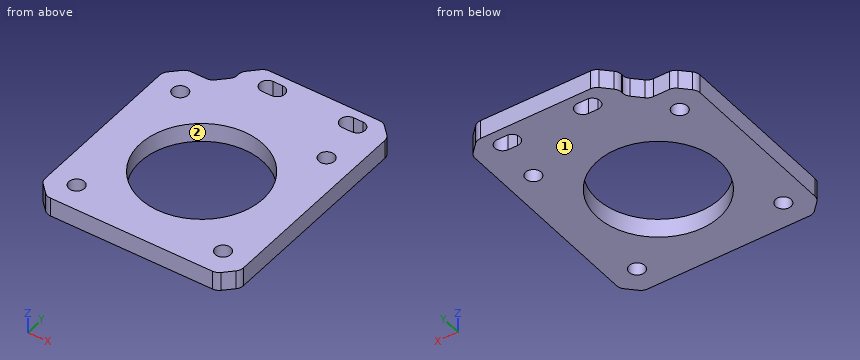
from build123d import *

# Parameters (mm, degrees)
SKETCH026_R     = 13
SKETCH026_R_2   = 1.65
PAD013_DEPTH    = 4
CHAMFER009_SIZE = 3
FILLET002_R     = 2


with BuildPart() as part:
    # Sketch026 → Pad013 (new body)
    with BuildSketch(Plane.XY):
        Polygon((-21, -21), (-21, 21), (-10, 21), (-10, 29), (21, 29), (21, -21), align=None)
        Circle(SKETCH026_R, mode=Mode.SUBTRACT)
        with Locations((-15.5, 15.5)):
            Circle(SKETCH026_R_2, mode=Mode.SUBTRACT)
        with Locations((15.5, 15.5)):
            Circle(SKETCH026_R_2, mode=Mode.SUBTRACT)
        with Locations((15.5, -15.5)):
            Circle(SKETCH026_R_2, mode=Mode.SUBTRACT)
        with Locations((-15.5, -15.5)):
            Circle(SKETCH026_R_2, mode=Mode.SUBTRACT)
        with BuildLine():
            ThreePointArc((-4, 27.05), (-5.65, 25.4), (-4, 23.75))
            Line((-4, 23.75), (-2, 23.75))
            ThreePointArc((-2, 23.75), (-0.35, 25.4), (-2, 27.05))
            Line((-2, 27.05), (-4, 27.05))
        make_face(mode=Mode.SUBTRACT)
        with BuildLine():
            ThreePointArc((13, 27.05), (11.35, 25.4), (13, 23.75))
            Line((13, 23.75), (15, 23.75))
            ThreePointArc((15, 23.75), (16.65, 25.4), (15, 27.05))
            Line((15, 27.05), (13, 27.05))
        make_face(mode=Mode.SUBTRACT)
    extrude(amount=PAD013_DEPTH)

    # Chamfer009
    chamfer009_edges = [part.edges().sort_by_distance(p)[0] for p in [
        (-10, 29, 2),
        (-10, 21, 2),
        (21, 29, 2),
        (21, -21, 2),
        (-21, -21, 2),
        (-21, 21, 2),
    ]]
    chamfer(chamfer009_edges, length=CHAMFER009_SIZE)

    # Fillet002
    fillet002_edges = [part.edges().sort_by_distance(p)[0] for p in [
        (21, 26, 2),
        (18, 29, 2),
        (21, -18, 2),
        (18, -21, 2),
        (-18, -21, 2),
        (-21, -18, 2),
        (-18, 21, 2),
        (-21, 18, 2),
        (-13, 21, 2),
        (-10, 24, 2),
        (-10, 26, 2),
        (-7, 29, 2),
    ]]
    fillet(fillet002_edges, radius=FILLET002_R)


with BuildPart() as part_1:
    # Body011 placement: moved
    add(part.part.moved(Location((30, -32, 50))))


solid = part_1.part
The listing builds one solid part. Answer for the finished solid, in the listing's coordinates (mm). Face numbers are marked on the shaded views. Coordinates: 2 decimals unless noted, no trailing zeros. Write each loop counter-clockwise with the first axis right and the second up, starting at its lowest first coordinate (ties: lowest second). Pieces come first, ordered by that corner, then holes. Notation, with made-up numbers: (2.25, 56) -> (50.25, 56) arc R8 ccw to (50.25, 68) -> close; hole circle Ø7 at (57, 5.25). An arc over 180 degrees is marked (long way). One line per question, with ' | ' between items.
1. Straight lines are drawn through the part: line 1 (Y direction, x = 14.5, z = 53.1); line 2 (X direction, y = -15, z = 52.35); line 3 (X direction, y = -8, z = 50.65). For each, find the intervals that lie inside material, in ascending order.
Verdict:
line 1: y = -53 to -49.15, -45.85 to -18.15, -14.85 to -11 | line 2: x = 9 to 13.81, 15.19 to 44.81, 46.19 to 51 | line 3: x = 19.82 to 25.13, 28.87 to 42.13, 45.87 to 51
2. For a pull along X with two mould halves and no side action, classify the marked faces 1 and 2 as released by +X, released by -X, zero draft, split by the parting line, or undercut.
Verdict:
face 1: zero draft | face 2: undercut
3. Section B-B (x = 14.5) is taken. Determine the outline of the cut face in (y, z), and give its area (3 significant figures).
Verdict:
outline: (-53, 50) -> (-49.15, 50) -> (-49.15, 54) -> (-53, 54) -> close; (-45.85, 50) -> (-18.15, 50) -> (-18.15, 54) -> (-45.85, 54) -> close; (-14.85, 50) -> (-11, 50) -> (-11, 54) -> (-14.85, 54) -> close | area: 142 mm^2
4. Section D-D (z = 53.35) is taken. State how many separate pieces and enclosed holes the cut face has, and give its area (3 significant figures).
Verdict:
separate pieces: 1 | enclosed holes: 7 | area: 1,400 mm^2
5. Section C-C (x = 31.5) is taken. Determine the outline of the cut face in (y, z).
Verdict:
outline: (-53, 50) -> (-44.91, 50) -> (-44.91, 54) -> (-53, 54) -> close; (-19.09, 50) -> (-3, 50) -> (-3, 54) -> (-19.09, 54) -> close
6. Section A-A (y = -32) is taken. Determine the outline of the cut face in (x, z), and give its area (3 significant figures).
Verdict:
outline: (9, 50) -> (17, 50) -> (17, 54) -> (9, 54) -> close; (43, 50) -> (51, 50) -> (51, 54) -> (43, 54) -> close | area: 64.0 mm^2
